from build123d import *

# Parameters (mm, degrees)
SKETCH1_R           = 13.45
BOSS_EXTRUDE2_DEPTH = 48
SKETCH7_W           = 44
SKETCH7_H           = 14
SKETCH7_R           = 4.5
SKETCH7_R_2         = 4.1
BOSS_EXTRUDE3_DEPTH = 13
FILLET1_R           = 3
FILLET2_R           = 5
FILLET3_R           = 5
FILLET4_R           = 3
SKETCH8_R           = 4.1
SKETCH8_R_2         = 4.5
CUT_EXTRUDE1_DEPTH  = 192.299242027


with BuildPart() as part:
    # Sketch1 → Boss-Extrude2 (new body)
    with BuildSketch(Plane(origin=(0, 0, 0), x_dir=(1, 0, 0), z_dir=(0, 1, 0))):
        Polygon((-17.4, 17.4), (17.4, 17.4), (17.4, -17.4), (-17.4, -17.4), (-17.4, 13.4), (-82.6, 13.4), (-82.6, 17.4), align=None)
        with Locations(Location((0, 0, 0), (0, 0, 270))):
            Circle(SKETCH1_R, mode=Mode.SUBTRACT)
    boss_extrude2 = extrude(amount=BOSS_EXTRUDE2_DEPTH)

    # Mirror2: Boss-Extrude2 across plane
    add(boss_extrude2.mirror(Plane(origin=(-82.6, 48, -17.4), x_dir=(0, 0, 1), z_dir=(1, 0, 0))))

    # Sketch7 → Boss-Extrude3 (add)
    with BuildSketch(Plane.XY.offset(-13.4)):
        with Locations((-97.6, 24)):
            Rectangle(SKETCH7_W, SKETCH7_H)
        with Locations(Location((-82.6, 24, 0), (0, 0, 180))):
            Circle(SKETCH7_R, mode=Mode.SUBTRACT)
        with Locations(Location((-112.6, 24, 0), (0, 0, 180))):
            Circle(SKETCH7_R_2, mode=Mode.SUBTRACT)
    extrude(amount=BOSS_EXTRUDE3_DEPTH)

    # Fillet1
    fillet1_edges = [part.edges().sort_by_distance(p)[0] for p in [
        (17.4, 24, 17.4),
        (-17.4, 24, 17.4),
        (-182.6, 24, 17.4),
        (-147.8, 24, 17.4),
    ]]
    fillet(fillet1_edges, radius=FILLET1_R)

    # Fillet2
    fillet2_edges = [part.edges().sort_by_distance(p)[0] for p in [
        (-17.4, 24, -13.4),
        (17.4, 24, -17.4),
        (-182.6, 24, -17.4),
        (-147.8, 24, -13.4),
    ]]
    fillet(fillet2_edges, radius=FILLET2_R)

    # Fillet3
    fillet3_edges = [part.edges().sort_by_distance(p)[0] for p in [
        (-75.6, 17, -6.9),
        (-75.6, 31, -6.9),
        (-119.6, 31, -6.9),
        (-119.6, 17, -6.9),
    ]]
    fillet(fillet3_edges, radius=FILLET3_R)

    # Fillet4
    fillet4_edges = [part.edges().sort_by_distance(p)[0] for p in [
        (-97.6, 31, -13.4),
        (-75.6, 24, -13.4),
        (-97.6, 17, -13.4),
        (-119.6, 24, -13.4),
        (-77.064466094, 29.535533906, -13.4),
        (-77.064466094, 18.464466094, -13.4),
        (-118.135533906, 29.535533906, -13.4),
        (-118.135533906, 18.464466094, -13.4),
    ]]
    fillet(fillet4_edges, radius=FILLET4_R)

    # Sketch8 → Cut-Extrude1 (cut, through all)
    with BuildSketch(Plane.XY.offset(-13.4)):
        with Locations(Location((-112.6, 24, 0), (0, 0, 180))):
            Circle(SKETCH8_R)
        with Locations(Location((-82.6, 24, 0), (0, 0, 180))):
            Circle(SKETCH8_R_2)
    extrude(amount=-CUT_EXTRUDE1_DEPTH, mode=Mode.SUBTRACT)


solid = part.part
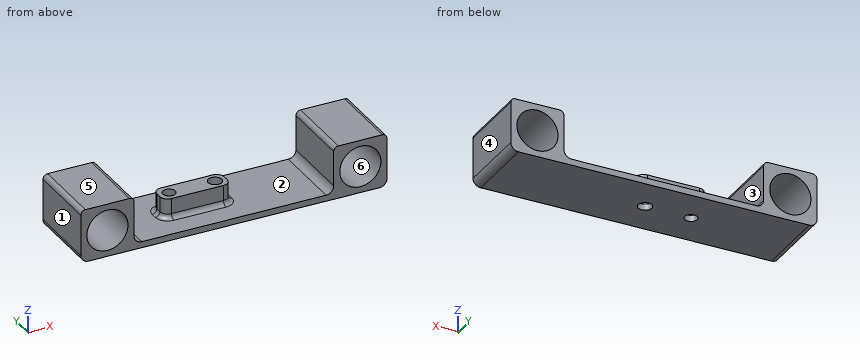
Can you work these out from the model? Positions are in its coordinate system, mm. Face numbers are marked on the shaded views. A direction names the side the tool comes from. Give positions to 0.01 mm unless a question says otherwise; leave off trailing zeros. Write each loop counter-clockwise with the first axis right and the second up, starting at its lowest first coordinate (ties: lowest second). Pieces come first, ordered by that corner, then holes. Notation, with made-up numbers: (70, 85.25) -> (88, 85.25) arc R21 ccw to (88, 106.25) -> close; hole circle Ø4 at (-25.75, 35.5). An arc over 180 degrees is marked (long way). Answer as a JSON object with one key per item and string values. Group by question number.
Item 1: Suppose I cut it at D-D (y = 43). Please give me the cut outline in (x, z).
Item 2: Suppose I cut it at C-C (z = -4.5). Please give me the cut outline in (x, y), plus the area to 3 significant figures.
Item 3: I'm going to push flat-ended pins straight in: P1, Ø24, axis at x = -82.5, y = 13.5, coming from the +Z side; P2, Ø5.5, axis at x = -82.6, y = 24, coming from the +Z side; P3, Ø11, axis at x = -94.5, z = -4, coming from the -Y side; P4, Ø10, axis at x = -135, y = 30.5, coming from the +Z side. Where does each tip first touch, or does it pass through?
Item 4: We'd pull the mould along Z, two halves only. Please class the marked faces 4, 5 and 6: +Z half, -Z half, draft (parallel to the pull), parting line (faces both ways), or undercut.
Item 5: Suppose I cut it at A-A (y = 24). State how many separate pieces and enclosed holes the cut face has, plus the area to 3 significant figures.
Item 6: Suppose I cut it at B-B (x = -165.2). Please give me the cut outline in (y, z), plus the area to 3 significant figures.
Item 7: Please list where these lines run through material, in increasing order: line 1 (X direction, y = 13, z = 0); line 2 (Y direction, x = -82.6, z = -4.5); line 3 (Z direction, x = -165.2, y = 23.5). Write a range as [from, to].
Item 8: For the marked faces 1, 2 and 3, which set-ups out of +Z, -Z, +X, -X, +Y, -Y let a thin tool reach every point of the face, with its end or its side?
Findings:
{
 "1": {"outline": "(-182.6, -12.4) arc R5 ccw to (-177.6, -17.4) -> (12.4, -17.4) arc R5 ccw to (17.4, -12.4) -> (17.4, 14.4) arc R3 ccw to (14.4, 17.4) -> (-14.4, 17.4) arc R3 ccw to (-17.4, 14.4) -> (-17.4, -8.4) arc R5 cw to (-22.4, -13.4) -> (-142.8, -13.4) arc R5 cw to (-147.8, -8.4) -> (-147.8, 14.4) arc R3 ccw to (-150.8, 17.4) -> (-179.6, 17.4) arc R3 ccw to (-182.6, 14.4) -> close; hole circle Ø26.9 at (-165.2, 0); hole circle Ø26.9 at (0, 0)"},
 "2": {"outline": "(-182.6, 0) -> (-177.87, 0) -> (-177.87, 48) -> (-182.6, 48) -> close; (-152.53, 0) -> (-147.8, 0) -> (-147.8, 48) -> (-152.53, 48) -> close; (-119.6, 22) arc R5 ccw to (-114.6, 17) -> (-80.6, 17) arc R5 ccw to (-75.6, 22) -> (-75.6, 26) arc R5 ccw to (-80.6, 31) -> (-114.6, 31) arc R5 ccw to (-119.6, 26) -> close; (-17.4, 0) -> (-12.67, 0) -> (-12.67, 48) -> (-17.4, 48) -> close; (12.67, 0) -> (17.4, 0) -> (17.4, 48) -> (12.67, 48) -> close; hole circle Ø8.2 at (-112.6, 24); hole circle Ø9 at (-82.6, 24)", "area": "1,390 mm²"},
 "3": {"P1": "stops at z = -0.4", "P2": "passes through", "P3": "stops at y = 17", "P4": "stops at z = -13.4"},
 "4": {"face 4": "draft", "face 5": "+Z half", "face 6": "undercut"},
 "5": {"separate pieces": "3", "enclosed holes": "2", "area": "2,080 mm²"},
 "6": {"outline": "(0, -17.4) -> (48, -17.4) -> (48, -13.45) -> (0, -13.45) -> close; (0, 13.45) -> (48, 13.45) -> (48, 17.4) -> (0, 17.4) -> close", "area": "379 mm²"},
 "7": {"line 1": "x = [-182.6, -178.65], [-151.75, -147.8], [-17.4, -13.45], [13.45, 17.4]", "line 2": "y = [17, 19.5], [28.5, 31]", "line 3": "z = [-17.4, -13.45], [13.45, 17.4]"},
 "8": {"face 1": "+Z, -Z, -X, +Y, -Y", "face 2": "+Z", "face 3": "+Z, +Y, -Y"}
}
